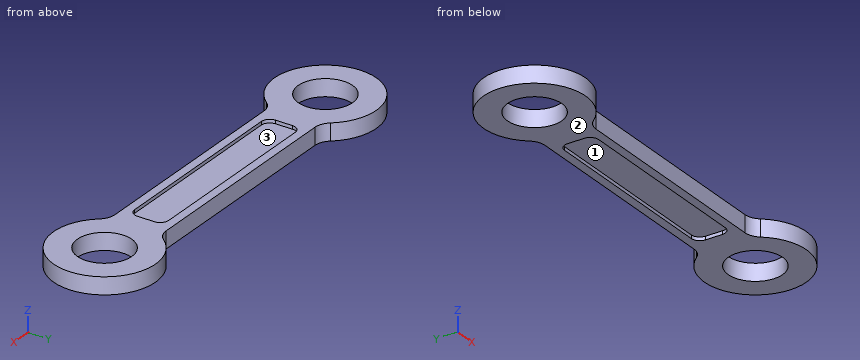
```python
from build123d import *

# Parameters (mm, degrees)
BOSS_EXTRUDE1_DEPTH      = 5
BOSS_EXTRUDE1_DEPTH_BACK = 5
SKETCH1_R                = 16
FILLET1_R                = 10
CUT_EXTRUDE1_DEPTH       = 2


with BuildPart() as part:
    # Sketch1 → Boss-Extrude1 (new, two sides: drawn at the far end of the back side and taken through both)
    with BuildSketch(Plane.XY.offset(-BOSS_EXTRUDE1_DEPTH_BACK)):
        with BuildLine():
            Line((-70, -15), (70, -15))
            ThreePointArc((70, -15), (125.980762114, 0), (70, 15))
            Line((70, 15), (-70, 15))
            ThreePointArc((-70, 15), (-125.980762114, 0), (-70, -15))
        make_face()
        with Locations((-95.980762114, 0)):
            Circle(SKETCH1_R, mode=Mode.SUBTRACT)
        with Locations((95.980762114, 0)):
            Circle(SKETCH1_R, mode=Mode.SUBTRACT)
    extrude(amount=BOSS_EXTRUDE1_DEPTH + BOSS_EXTRUDE1_DEPTH_BACK)

    # Fillet1
    fillet1_edges = [part.edges().sort_by_distance(p)[0] for p in [
        (70, -15, 0),
        (-70, -15, 0),
        (-70, 15, 0),
        (70, 15, 0),
    ]]
    fillet(fillet1_edges, radius=FILLET1_R)

    # Sketch2 → Cut-Extrude1 (cut)
    with BuildSketch(Plane.XY.offset(5)):
        with BuildLine():
            Line((55, 10), (-55, 10))
            ThreePointArc((-55, 10), (-58.535533906, 8.535533906), (-60, 5))
            Line((-60, 5), (-60, -5))
            ThreePointArc((-60, -5), (-58.535533906, -8.535533906), (-55, -10))
            Line((-55, -10), (55, -10))
            ThreePointArc((55, -10), (58.535533906, -8.535533906), (60, -5))
            Line((60, -5), (60, 5))
            ThreePointArc((60, 5), (58.535533906, 8.535533906), (55, 10))
        make_face()
    cut_extrude1 = extrude(amount=-CUT_EXTRUDE1_DEPTH, mode=Mode.SUBTRACT)

    # Mirror4: Cut-Extrude1 across plane
    add(cut_extrude1.mirror(Plane.XY), mode=Mode.SUBTRACT)


solid = part.part
```
Input: part model. Units: mm. Frame: model coordinates. Face numbers are marked on the shaded views. Coordinates: 2 decimals unless noted, no trailing zeros. Order: outer loops, then holes, each group sorted by start corner. A loop starts at its lowest first (then second) coordinate and runs counter-clockwise, first axis right, second up. Notation, with made-up numbers: (21.5, 10) - (54.5, 10) arc R14 cw to (54.5, 21) - close; hole circle Ø3 at (-24, 73.5). An arc over 180 degrees is marked (long way). Return JSON: item names as keys, results as strings.
Q1. Ray query, probe 1 along X at (y, z) = (-2, 1.25); probe 2 along X at (y, z) = (-11, 2.25); probe 3 along Y at (x, z) = (51, 3.5). Return the intervals inside material, ascending.
The answers:
{"probe 1": "x = -125.91 to -111.86, -80.11 to 80.11, 111.86 to 125.91", "probe 2": "x = -123.89 to -107.6, -84.36 to 84.36, 107.6 to 123.89", "probe 3": "y = -15 to -10, 10 to 15"}
Q2. Cut plane C-C (x = 43). Return loops of the section in (y, z).
The answers:
{"outline": "(-15, -5) - (-10, -5) - (-10, -3) - (10, -3) - (10, -5) - (15, -5) - (15, 5) - (10, 5) - (10, 3) - (-10, 3) - (-10, 5) - (-15, 5) - close"}
Q3. Cut plane A-A (z = -0.75). Return loops of the section in (x, y).
The answers:
{"outline": "(-72.56, -18.75) arc R10 cw to (-64.76, -15) - (64.76, -15) arc R10 cw to (72.56, -18.75) arc R30 ccw (long way) to (72.56, 18.75) arc R10 cw to (64.76, 15) - (-64.76, 15) arc R10 cw to (-72.56, 18.75) arc R30 ccw (long way) to start; hole circle Ø32 at (-95.98, 0); hole circle Ø32 at (95.98, 0)"}
Q4. Draft query along X for the marked faces 1, 2 and 3. Return one class per face: +X half, -X half, draft (parallel to the pull), parting line (faces both ways), or undercut.
The answers:
{"face 1": "undercut", "face 2": "draft", "face 3": "undercut"}
Q5. Cut plane B-B (y = 2.5). Return loops of the section in (x, z).
The answers:
{"outline": "(-125.88, -5) - (-111.78, -5) - (-111.78, 5) - (-125.88, 5) - close; (-80.18, -5) - (-60, -5) - (-60, -3) - (60, -3) - (60, -5) - (80.18, -5) - (80.18, 5) - (60, 5) - (60, 3) - (-60, 3) - (-60, 5) - (-80.18, 5) - close; (111.78, -5) - (125.88, -5) - (125.88, 5) - (111.78, 5) - close"}
Q6. First-contact query: pin 1 (4 mm diameter, centred on x = -67.5, z = -2.5, fed in from -Y); pin 2 (2 mm diameter, centred on x = 23, z = 4, fed in from -Y); pin 3 (10 mm diameter, centred on x = -22.5, y = 3.5, fed in from +Z). Flat tips, straight axial feed; report the tip coordinate or a pass-through.
The answers:
{"pin 1": "stops at y = -16.2", "pin 2": "stops at y = -15", "pin 3": "stops at z = 3"}
